```python
from build123d import *

# Parameters (mm, degrees)
CYLINDER001_R               = 1.2
CYLINDER001_DEPTH           = 10
CYLINDER001_ROLL_ANGLE      = -45
CYLINDER001_PLACEMENT_ANGLE = 45
CYLINDER002_R               = 1.2
CYLINDER002_DEPTH           = 10
CYLINDER002_ROLL_ANGLE      = 45
CYLINDER002_PLACEMENT_ANGLE = -45
CYLINDER003_R               = 1.2
CYLINDER003_DEPTH           = 10
CYLINDER003_ROLL_ANGLE      = 45
CYLINDER003_PLACEMENT_ANGLE = 45
CYLINDER_R                  = 1.2
CYLINDER_DEPTH              = 10
CYLINDER_ROLL_ANGLE         = -45
CYLINDER_PLACEMENT_ANGLE    = -45
PAD_DEPTH                   = 5
SKETCH003_R                 = 0.9
POCKET001_DEPTH             = 7.001
SKETCH001_R                 = 1.2
POCKET_DEPTH                = 38.001


with BuildPart() as cylinder001:
    # Cylinder001 → Cylinder001 (new body)
    with BuildSketch(Plane.XY):
        Circle(CYLINDER001_R)
    extrude(amount=CYLINDER001_DEPTH)


with BuildPart() as cylinder001_1:
    # Cylinder001 roll: moved
    add(cylinder001.part.rotate(Axis((0, 0, 0), (1, 0, 0)), CYLINDER001_ROLL_ANGLE))


with BuildPart() as cylinder001_2:
    # Cylinder001 placement: moved
    add(cylinder001_1.part.moved(Location((14.349242, -14.349242, 7.292893))).rotate(Axis((14.349242, -14.349242, 7.292893), (0, 0, 1)), CYLINDER001_PLACEMENT_ANGLE))


with BuildPart() as cylinder002:
    # Cylinder002 → Cylinder002 (new body)
    with BuildSketch(Plane.XY):
        Circle(CYLINDER002_R)
    extrude(amount=CYLINDER002_DEPTH)


with BuildPart() as cylinder002_1:
    # Cylinder002 roll: moved
    add(cylinder002.part.rotate(Axis((0, 0, 0), (1, 0, 0)), CYLINDER002_ROLL_ANGLE))


with BuildPart() as cylinder002_2:
    # Cylinder002 placement: moved
    add(cylinder002_1.part.moved(Location((14.349242, 14.349242, 7.292893))).rotate(Axis((14.349242, 14.349242, 7.292893), (0, 0, 1)), CYLINDER002_PLACEMENT_ANGLE))


with BuildPart() as cylinder003:
    # Cylinder003 → Cylinder003 (new body)
    with BuildSketch(Plane.XY):
        Circle(CYLINDER003_R)
    extrude(amount=CYLINDER003_DEPTH)


with BuildPart() as cylinder003_1:
    # Cylinder003 roll: moved
    add(cylinder003.part.rotate(Axis((0, 0, 0), (1, 0, 0)), CYLINDER003_ROLL_ANGLE))


with BuildPart() as cylinder003_2:
    # Cylinder003 placement: moved
    add(cylinder003_1.part.moved(Location((-14.349242, 14.349242, 7.292893))).rotate(Axis((-14.349242, 14.349242, 7.292893), (0, 0, 1)), CYLINDER003_PLACEMENT_ANGLE))


with BuildPart() as fusion001:
    # Cylinder → Cylinder (new body)
    with BuildSketch(Plane.XY):
        Circle(CYLINDER_R)
    extrude(amount=CYLINDER_DEPTH)


with BuildPart() as fusion001_1:
    # Cylinder roll: moved
    add(fusion001.part.rotate(Axis((0, 0, 0), (1, 0, 0)), CYLINDER_ROLL_ANGLE))


with BuildPart() as fusion001_2:
    # Cylinder placement: moved
    add(fusion001_1.part.moved(Location((-14.349242, -14.349242, 7.292893))).rotate(Axis((-14.349242, -14.349242, 7.292893), (0, 0, 1)), CYLINDER_PLACEMENT_ANGLE))

    # Fusion001: union Cylinder001, Cylinder002, Cylinder003
    add(cylinder001_2.part)
    add(cylinder002_2.part)
    add(cylinder003_2.part)


with BuildPart() as body001:
    # Sketch002 → Pad (new body)
    with BuildSketch(Plane.YZ):
        Polygon((14, 10), (14, 35), (16, 35), (16, 25), (19, 25), (19, 35), (21, 35), (21, 10), align=None)
    extrude(amount=PAD_DEPTH)

    # Sketch003 (on Face1 of Pad) → Pocket001 (cut, through all)
    with BuildSketch(Plane(origin=(0, 14, 0), x_dir=(0, 0, -1), z_dir=(0, -1, 0))):
        with Locations((-31, 2.5)):
            Circle(SKETCH003_R)
    extrude(amount=-POCKET001_DEPTH, mode=Mode.SUBTRACT)


with BuildPart() as body001_1:
    # Body001 placement: moved
    add(body001.part.moved(Location((-2.5, 0, 0))))


with BuildPart() as cut:
    # Sketch → Revolution (revolve)
    with BuildSketch(Plane.XZ):
        Polygon((16, 4), (16, 0), (14, 0), (14, 10), (21, 10), align=None)
    revolve(axis=Axis((0, 0, 0), (0, 0, 1)))

    # Sketch001 → Pocket (cut, through all)
    with BuildSketch(Plane.XZ.offset(17)):
        with Locations((0, 2)):
            Circle(SKETCH001_R)
    extrude(amount=-POCKET_DEPTH, mode=Mode.SUBTRACT)

    # Fusion: union Body001
    add(body001_1.part)

    # Cut: cut Fusion001
    add(fusion001_2.part, mode=Mode.SUBTRACT)


solid = cut.part
```
The listing builds one solid part. Answer for the finished solid, in the listing's coordinates (mm). A direction names the side the tool comes from. Coordinates: 2 decimals unless noted, no trailing zeros. Write each loop counter-clockwise with the first axis right and the second up, starting at its lowest first coordinate (ties: lowest second). Pieces come first, ordered by that corner, then holes.
Q1. Section D-D, the plane z = 14.5 is taken. Write down the section's boundary in (x, y), then the cut area to 3 significant figures.
Returned:
outline: (-2.5, 14) - (2.5, 14) - (2.5, 21) - (-2.5, 21) - close
area: 35.0 mm2
Q2. Which of the six approach directions +Z, -Z, +X, -X, +Y, -Y give full straight-line access (tool end or side, diameter ignored) to faces 1 (the flat face through (-2.5, 18, 23)), 2 (the flat face through (2.5, 18, 23)), 3 (the flat face through (0, 17, 25)), 4 (the flat face through (0, 14, 22)), 5 (the flat face through (0, 21, 23))?
Returned:
face 1: +Z, -X, +Y, -Y
face 2: +Z, +X, +Y, -Y
face 3: +Z, +X, -X
face 4: +Z, +X, -X, -Y
face 5: +Z, -Z, +X, -X, +Y
Q3. The mould has two halves that part along X. Classify faces 6 (the flat face through (-0.07, -14.15, 0)), 7 (the cylindrical face through (-12.65, 12.28, 8.3)), 8 (the cylindrical face through (-3.47, -15.62, 1.97)): released by +X, released by -X, zero draft, split by the parting line, or undercut.
Returned:
face 6: zero draft
face 7: undercut
face 8: split by the parting line
Q4. Find the intervals of material crossed by line 1 along X through (y, z) = (20, 31); line 2 along Y through (x, z) = (0, 3.75); line 3 along Z through (x, y) = (0, -15.1), in increasing order.
Returned:
line 1: x = -2.5 to -0.9, 0.9 to 2.5
line 2: y = -16 to -14, 14 to 16
line 3: z = 0 to 0.8, 3.2 to 10
Q5. Section A-A, the plane y = 0 is taken. Write down the section's boundary in (x, z), then the cut area to 3 significant figures.
Returned:
outline: (-21, 10) - (-16, 4) - (-16, 0) - (-14, 0) - (-14, 10) - close; (14, 0) - (16, 0) - (16, 4) - (21, 10) - (14, 10) - close
area: 70.0 mm2
Q6. Given P1, Ø3, axis at x = 0, z = 31, coming from the +Y side; P2, Ø7.5, axis at y = 18, z = 26.5, coming from the -X side; P3, Ø5.5, axis at x = 0.5, z = 23.5, coming from the -Y side; P4, Ø1, axis at x = 16.5, y = 11.5, coming from the +Z side, each flat-ended and moving along its own axis, determine where each tip first touches the part or whether it passes through.
Returned:
P1: stops at y = 21
P2: stops at x = -2.5
P3: stops at y = 14
P4: stops at z = 10
Q7. Section B-B, the plane z = 31 is taken. Write down the section's boundary in (x, y), then the cut area to 3 significant figures.
Returned:
outline: (-2.5, 14) - (-0.9, 14) - (-0.9, 16) - (-2.5, 16) - close; (-2.5, 19) - (-0.9, 19) - (-0.9, 21) - (-2.5, 21) - close; (0.9, 14) - (2.5, 14) - (2.5, 16) - (0.9, 16) - close; (0.9, 19) - (2.5, 19) - (2.5, 21) - (0.9, 21) - close
area: 12.8 mm2
